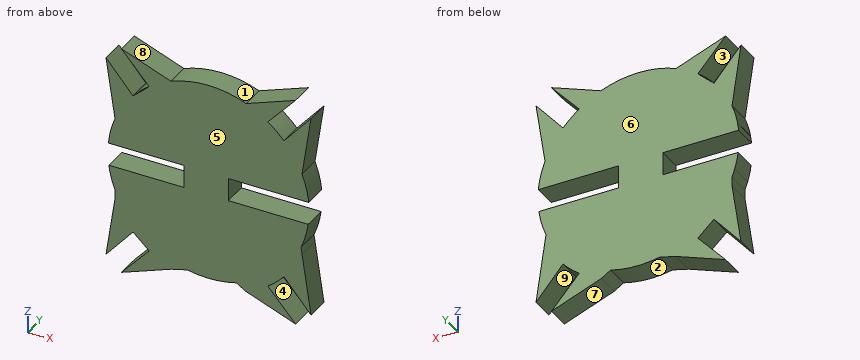
```python
from build123d import *

# Parameters (mm, degrees)
F1_DEPTH = 4.3434


with BuildPart() as f1:
    # F0 (on Front) → F1 (new body)
    with BuildSketch(Plane.XZ):
        with BuildLine():
            ThreePointArc((15.940657, -30.021235), (15.833766, -30.712775), (15.753128, -31.407866))
            Line((15.753128, -31.407866), (15.761479, -31.407866))
            ThreePointArc((15.761479, -31.407866), (15.837097, -30.743943), (15.936717, -30.083195))
            Line((15.936717, -30.083195), (15.940657, -30.021235))
        make_face()
        with BuildLine():
            ThreePointArc((15.936717, -30.083195), (15.837097, -30.743943), (15.761479, -31.407866))
            Line((15.761479, -31.407866), (29.639391, -31.407866))
            Line((29.639391, -31.407866), (29.639391, -34.026345))
            Line((29.639391, -34.026345), (37.738703, -34.026345))
            Line((37.738703, -34.026345), (37.738703, -33.516066))
            Line((37.738703, -33.516066), (37.738703, -31.407866))
            Line((37.738703, -31.407866), (52.500848, -31.407866))
            ThreePointArc((52.500848, -31.407866), (52.059884, -28.853474), (51.265883, -26.385899))
            Line((51.265883, -26.385899), (52.917353, -15.238802))
            Line((52.917353, -15.238802), (47.958307, -21.024324))
            ThreePointArc((47.958307, -21.024324), (46.547291, -19.593445), (44.989268, -18.324217))
            Line((44.989268, -18.324217), (50.081812, -12.655849))
            Line((50.081812, -12.655849), (41.014464, -16.056665))
            Line((41.014464, -16.056665), (40.930312, -16.088227))
            ThreePointArc((40.930312, -16.088227), (34.112246, -14.784679), (27.294179, -16.088227))
            Line((27.294179, -16.088227), (27.21875, -16.059937))
            Line((27.21875, -16.059937), (18.142679, -12.655849))
            Line((18.142679, -12.655849), (23.20848, -18.294449))
            Line((23.20848, -18.294449), (23.235223, -18.324217))
            Line((23.235223, -18.324217), (20.266184, -21.024324))
            Line((20.266184, -21.024324), (20.25096, -21.006563))
            Line((20.25096, -21.006563), (15.307139, -15.238802))
            Line((15.307139, -15.238802), (16.958609, -26.385899))
            ThreePointArc((16.958609, -26.385899), (16.344763, -28.176471), (15.917278, -30.020437))
            Line((15.917278, -30.020437), (15.940657, -30.021235))
            Line((15.940657, -30.021235), (15.936717, -30.083195))
        make_face()
        with BuildLine():
            Line((37.738703, -34.026345), (29.639391, -34.026345))
            Line((29.639391, -34.026345), (29.639391, -35.624266))
            Line((29.639391, -35.624266), (15.82806, -35.624266))
            ThreePointArc((15.82806, -35.624266), (16.090138, -37.12187), (16.474419, -38.592866))
            ThreePointArc((16.474419, -38.592866), (16.702769, -39.290058), (16.958609, -39.977639))
            Line((16.958609, -39.977639), (16.958609, -41.666792))
            Line((16.958609, -41.666792), (15.307139, -52.813889))
            Line((15.307139, -52.813889), (20.266184, -47.028366))
            Line((20.266184, -47.028366), (23.235223, -49.728474))
            Line((23.235223, -49.728474), (18.142679, -55.396842))
            Line((18.142679, -55.396842), (27.294179, -51.964463))
            Line((27.294179, -51.964463), (30.11443, -51.22633))
            Line((30.11443, -51.22633), (30.241821, -51.192989))
            ThreePointArc((30.241821, -51.192989), (34.753518, -51.594634), (39.227042, -50.884485))
            Line((39.227042, -50.884485), (40.930312, -51.964463))
            Line((40.930312, -51.964463), (50.081812, -55.396842))
            Line((50.081812, -55.396842), (44.989268, -49.728474))
            ThreePointArc((44.989268, -49.728474), (46.547291, -48.459245), (47.958307, -47.028366))
            Line((47.958307, -47.028366), (52.917353, -52.813889))
            Line((52.917353, -52.813889), (51.265883, -41.666792))
            Line((51.265883, -41.666792), (51.084311, -40.441218))
            Line((51.084311, -40.441218), (51.079733, -40.410318))
            ThreePointArc((51.079733, -40.410318), (51.90089, -38.061868), (52.398499, -35.624266))
            Line((52.398499, -35.624266), (37.738703, -35.624266))
            Line((37.738703, -35.624266), (37.738703, -34.026345))
        make_face()
        with BuildLine():
            ThreePointArc((21.213653, -19.98888), (20.72264, -20.488578), (20.25096, -21.006563))
            Line((20.25096, -21.006563), (20.266184, -21.024324))
            ThreePointArc((20.266184, -21.024324), (21.6772, -19.593445), (23.235223, -18.324217))
            Line((23.235223, -18.324217), (23.20848, -18.294449))
            ThreePointArc((23.20848, -18.294449), (22.18097, -19.106233), (21.213653, -19.98888))
        make_face()
        with BuildLine():
            ThreePointArc((51.084311, -40.441218), (51.904816, -38.077325), (52.398499, -35.624266))
            ThreePointArc((52.398499, -35.624266), (51.90089, -38.061868), (51.079733, -40.410318))
            Line((51.079733, -40.410318), (51.084311, -40.441218))
        make_face()
        with BuildLine():
            ThreePointArc((41.014464, -16.056665), (34.11629, -14.719787), (27.21875, -16.059937))
            Line((27.21875, -16.059937), (27.294179, -16.088227))
            ThreePointArc((27.294179, -16.088227), (34.112246, -14.784679), (40.930312, -16.088227))
            Line((40.930312, -16.088227), (41.014464, -16.056665))
        make_face()
    extrude(amount=F1_DEPTH)


solid = f1.part
```
Part model, mm, in its own coordinate system. Face numbers are marked on the shaded views. A direction names the side the tool comes from. Round coordinates to 2 decimals unless told otherwise and drop trailing zeros. Loops run counter-clockwise (first coordinate to the right, second up) from the corner with the lowest first, then second, coordinate; pieces in that order, holes last. Notation, with made-up numbers: (70, 36) -> (120, 36) arc R33 ccw to (120, 71) -> close; hole circle Ø10 at (59.25, -37.5). An arc over 180 degrees is marked (long way). Use a Markdown table: item, result.
1) Pull direction Z, two halves, no side cores. Call the marked faces 1, 2, 3 and 4: pulls with the +Z half, pulls with the -Z half, needs draft (parallel to the pull), parting line crosses it, or undercut.
The answers:
| item | result |
|---|---|
| face 1 | pulls with the +Z half |
| face 2 | pulls with the -Z half |
| face 3 | undercut |
| face 4 | undercut |
2) Cut at A-A, the plane x = 44.5. List the corners of the cut face in (y, z).
The answers:
| item | result |
|---|---|
| outline | (-4.34, -53.3) -> (0, -53.3) -> (0, -35.62) -> (-4.34, -35.62) -> close; (-4.34, -31.41) -> (0, -31.41) -> (0, -14.75) -> (-4.34, -14.75) -> close |
3) Tool access for the marked faces 5, 6, 7, 8 and 9: list every direction of +Z, -Z, +X, -X, +Y, -Y with a clear straight run to the whole face (end or side of a thin tool).
The answers:
| item | result |
|---|---|
| face 5 | +Z, -Z, +X, -X, -Y |
| face 6 | +Z, -Z, +X, -X, +Y |
| face 7 | -Z, +Y, -Y |
| face 8 | +Z, +Y, -Y |
| face 9 | +Y, -Y |
4) Cut at C-C, the plane x = 22.5. List the corners of the cut face in (y, z), and give its area (3 significant figures).
The answers:
| item | result |
|---|---|
| outline | (-4.34, -53.76) -> (0, -53.76) -> (0, -50.55) -> (-4.34, -50.55) -> close; (-4.34, -49.06) -> (0, -49.06) -> (0, -35.62) -> (-4.34, -35.62) -> close; (-4.34, -31.41) -> (0, -31.41) -> (0, -18.99) -> (-4.34, -18.99) -> close; (-4.34, -18.89) -> (0, -18.89) -> (0, -18.84) -> (-4.34, -18.84) -> close; (-4.34, -17.51) -> (0, -17.51) -> (0, -14.29) -> (-4.34, -14.29) -> close |
| area | 140 mm2 |
5) Drop flat-ended pins along their axis: pin 1 Ø1.5 at (y, z) = (-1.5, -48.5) entering from -X; pin 2 Ø1.5 at (y, z) = (-3, -23) entering from +X; pin 3 Ø2 at (x, y) = (34.5, -2) entering from +Z. Give the stop position or say it passes through.
The answers:
| item | result |
|---|---|
| pin 1 | stops at x = 15.84 |
| pin 2 | stops at x = 51.88 |
| pin 3 | stops at z = -14.72 |
6) Cut at B-B, the plane z = -17.5. List the corners of the cut face in (x, y).
The answers:
| item | result |
|---|---|
| outline | (15.64, -4.34) -> (17.25, -4.34) -> (17.25, 0) -> (15.64, 0) -> close; (22.49, -4.34) -> (45.73, -4.34) -> (45.73, 0) -> (22.49, 0) -> close; (50.98, -4.34) -> (52.58, -4.34) -> (52.58, 0) -> (50.98, 0) -> close |
7) Cut at D-D, the plane z = -34. List the corners of the cut face in (x, y), and give its area (3 significant figures).
The answers:
| item | result |
|---|---|
| outline | (29.64, -4.34) -> (37.74, -4.34) -> (37.74, 0) -> (29.64, 0) -> close |
| area | 35.2 mm2 |
8) Probe line 1 (Z direction, x = 48, y = -1.8); line 2 (Z direction, x = 29.5, y = -2.35); line 3 (Z direction, x = 41.5, y = -3.55). List the from-to ranges inside material, lowest first. Write a range as [from, to].
The answers:
| item | result |
|---|---|
| line 1 | z = [-54.62, -53.08], [-47.08, -35.62], [-31.41, -20.98], [-14.97, -13.44] |
| line 2 | z = [-51.39, -35.62], [-31.41, -15.31] |
| line 3 | z = [-52.18, -35.62], [-31.41, -15.87] |
